```python
from build123d import *

# Parameters (mm, degrees)
SKETCH1_W           = 25.4
SKETCH1_H           = 75
SKETCH1_R           = 2.1
BOSS_EXTRUDE1_DEPTH = 5
SKETCH2_W           = 10
SKETCH2_H           = 10.2
BOSS_EXTRUDE2_DEPTH = 5


with BuildPart() as part:
    # Sketch1 → Boss-Extrude1 (new body)
    with BuildSketch(Plane.XY):
        Rectangle(SKETCH1_W, SKETCH1_H)
        with Locations((0, -12.5)):
            Circle(SKETCH1_R, mode=Mode.SUBTRACT)
        with Locations((0, 17.5)):
            Circle(SKETCH1_R, mode=Mode.SUBTRACT)
    extrude(amount=BOSS_EXTRUDE1_DEPTH)

    # Sketch2 → Boss-Extrude2 (add)
    with BuildSketch(Plane.XY.offset(5)):
        with Locations((0, -37.5)):
            Rectangle(SKETCH2_W, SKETCH2_H)
    extrude(amount=-BOSS_EXTRUDE2_DEPTH)


solid = part.part
```
Read the model definition and answer for the solid it produces. Units are mm, in the model's axes. A direction names the side the tool comes from. Coordinates: 2 decimals unless noted, no trailing zeros. Write each loop counter-clockwise with the first axis right and the second up, starting at its lowest first coordinate (ties: lowest second). Pieces come first, ordered by that corner, then holes. Notation, with made-up numbers: (80.25, 28) -> (88.25, 28) arc R19 ccw to (88.25, 48) -> close; hole circle Ø2 at (75, 64). An arc over 180 degrees is marked (long way). Answer as a JSON object with one key per item and string values.
Q1. Determine the mould class of faces 1 (the flat face through (0, 37.5, 2)), 2 (the flat face through (9, -37.5, 2)), 3 (the flat face through (-5, -40, 3)), 4 (the cylindrical face through (1.13, 19.27, 2.46)) for opening direction Y: pulls with the +Y half, pulls with the -Y half, needs draft (parallel to the pull), parting line crosses it, or undercut.
The answers:
{"face 1": "pulls with the +Y half", "face 2": "pulls with the -Y half", "face 3": "needs draft", "face 4": "undercut"}
Q2. Consider line 1 (Y direction, x = 0, z = 1.2); line 2 (Y direction, x = 0.5, z = 0.6); line 3 (Y direction, x = -11.5, z = 2.65). Determine where each line is inside the solid, lowest interval first. Write a range as [from, to].
The answers:
{"line 1": "y = [-42.6, -14.6], [-10.4, 15.4], [19.6, 37.5]", "line 2": "y = [-42.6, -14.54], [-10.46, 15.46], [19.54, 37.5]", "line 3": "y = [-37.5, 37.5]"}
Q3. The part is cut by section C-C on x = 0. Give the vertices of the cut face in (y, z).
The answers:
{"outline": "(-42.6, 0) -> (-14.6, 0) -> (-14.6, 5) -> (-42.6, 5) -> close; (-10.4, 0) -> (15.4, 0) -> (15.4, 5) -> (-10.4, 5) -> close; (19.6, 0) -> (37.5, 0) -> (37.5, 5) -> (19.6, 5) -> close"}
Q4. The part is cut by section A-A on z = 3.15. Give the vertices of the cut face in (x, y).
The answers:
{"outline": "(-12.7, -37.5) -> (-5, -37.5) -> (-5, -42.6) -> (5, -42.6) -> (5, -37.5) -> (12.7, -37.5) -> (12.7, 37.5) -> (-12.7, 37.5) -> close; hole circle Ø4.2 at (0, -12.5); hole circle Ø4.2 at (0, 17.5)"}
Q5. A tool of negligible diameter and unlimited length cuts with its end or side. For faces 5 (the flat face through (-9, -37.5, 2)), 6 (the flat face through (0, -2, 0)), 7 (the flat face through (5, -40, 3)), from which of +Z, -Z, +X, -X, +Y, -Y can it reach the whole face along a straight path? Write none if from no direction.
The answers:
{"face 5": "+Z, -Z, -X, -Y", "face 6": "-Z, +X, -X, +Y, -Y", "face 7": "+Z, -Z, +X, -Y"}
Q6. Flat-ended cylindrical pins translate along their axes: pin 1 Ø1.5 at (x, z) = (7.5, 2.5) entering from -Y; pin 2 Ø1.5 at (y, z) = (-40.5, 3) entering from -X. Find the tip coordinate at first contact, or state that the pin passes through.
The answers:
{"pin 1": "stops at y = -37.5", "pin 2": "stops at x = -5"}
Q7. The part is cut by section B-B on y = -12.5. Give the vertices of the cut face in (x, z), then the cut area to 3 significant figures.
The answers:
{"outline": "(-12.7, 0) -> (-2.1, 0) -> (-2.1, 5) -> (-12.7, 5) -> close; (2.1, 0) -> (12.7, 0) -> (12.7, 5) -> (2.1, 5) -> close", "area": "106 mm2"}
Q8. The part is cut by section D-D on x = 7.75. Give the vertices of the cut face in (y, z).
The answers:
{"outline": "(-37.5, 0) -> (37.5, 0) -> (37.5, 5) -> (-37.5, 5) -> close"}
